Read the model definition and answer for the solid it produces. Units are mm, in the model's axes. Face numbers are marked on the shaded views. A direction names the side the tool comes from. Give positions to 0.01 mm unless a question says otherwise; leave off trailing zeros. Loops run counter-clockwise (first coordinate to the right, second up) from the corner with the lowest first, then second, coordinate; pieces in that order, holes last.
(1) Find section B-B, the plane z = 4.5. Write down the section's boundary in (x, y).
(2) Straight lines are drawn through the part: probe 1 along X at (y, z) = (-3.75, -0.5); probe 2 along Z at (x, y) = (-9.5, -4); probe 3 along Y at (x, z) = (-8.5, -2.25). For each, find the intervals that lie inside material, in ascending order.
(3) Each of these flat-tipped pins is pushed along its axis until it touches: P1, Ø0.8, axis at x = -17.375, z = 7.375, coming from the +Y side (3 decimals); P2, Ø1.8, axis at x = -18, z = 7, coming from the -Y side; P3, Ø9, axis at x = 9, z = 0.5, coming from the +Y side; P4, Ø0.5, axis at y = -6.5, z = -8.5, coming from the -X side. Where does it stop, or does it pass through?
(4) Find section A-A, the plane x = -9. Write down the section's boundary in (y, z).
(5) Find section C-C, the plane y = -3.5. Write down the section's boundary in (x, z) (3 decimals).
(6) Determine the mould class of the marked faces 3, 4 and 5 for opening direction Z: pulls with the +Z half, pulls with the -Z half, needs draft (parallel to the pull), parting line crosses it, or undercut.
(7) Which of the six approach directions +Z, -Z, +X, -X, +Y, -Y give full straight-line access (tool end or side, diameter ignored) to the marked faces 1 and 2?
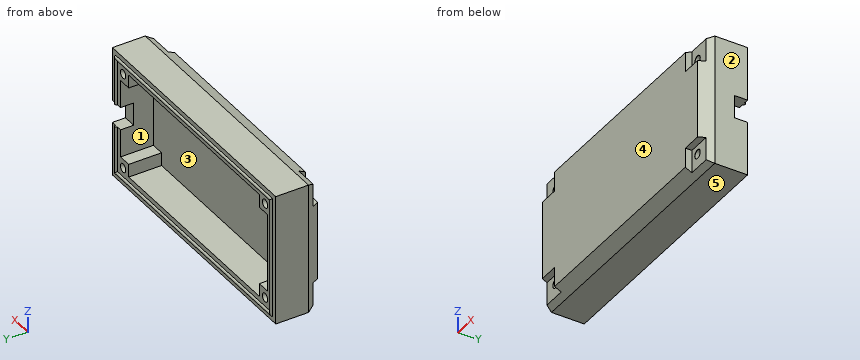
```python
from build123d import *

# Parameters (mm, degrees)
SCHIZZO2_W                     = 40
SCHIZZO2_H                     = 20
ESTRUSIONE_ESTRUSIONE1_DEPTH   = 7
TAGLIO_ESTRUSIONE1_DEPTH       = 5
SMUSSO1_SIZE                   = 1
SMUSSO1_SIZE2                  = 2
SCHIZZO6_W                     = 4
SCHIZZO6_H                     = 4
TAGLIO_ESTRUSIONE2_DEPTH       = 1
FORO_PER_VITE_M1_1_D           = 1.3
FORO_PER_VITE_M1_1_CSINK_D     = 1.35
FORO_PER_VITE_M1_1_CSINK_ANGLE = 90
SPECCHIA2_COPY_1_D             = 1.3
SPECCHIA2_COPY_1_CSINK_D       = 1.35
SPECCHIA2_COPY_1_CSINK_ANGLE   = 90
SCHIZZO14_W                    = 3.5
SCHIZZO14_H                    = 4
TAGLIO_ESTRUSIONE3_DEPTH       = 1
TAGLIO_ESTRUSIONE3_DEPTH_BACK  = 3


with BuildPart() as part:
    # Schizzo2 → Estrusione-Estrusione1 (new body)
    with BuildSketch(Plane(origin=(0, 0, 0), x_dir=(1, 0, 0), z_dir=(0, 1, 0))):
        Rectangle(SCHIZZO2_W, SCHIZZO2_H)
    extrude(amount=-ESTRUSIONE_ESTRUSIONE1_DEPTH)

    # Schizzo3 → Taglio-Estrusione1 (cut)
    with BuildSketch(Plane(origin=(0, 0, 0), x_dir=(1, 0, 0), z_dir=(0, 1, 0))):
        Polygon((-16, 8), (16, 8), (16, 6), (18, 6), (18, -6), (16, -6), (16, -8), (-16, -8), (-16, -6), (-18, -6), (-18, 6), (-16, 6), align=None)
    extrude(amount=-TAGLIO_ESTRUSIONE1_DEPTH, mode=Mode.SUBTRACT)

    # Sweep1: sweep along a path in Schizzo5
    with BuildLine(Plane(origin=(0, 0, 0), x_dir=(1, 0, 0), z_dir=(0, 1, 0))) as sweep1_path:
        Line((19, -9), (-19, -9))
        Line((-19, -9), (-19, 9))
        Line((-19, 9), (19, 9))
        Line((19, 9), (19, -9))
    # Schizzo4 → Sweep1 (sweep)
    with BuildSketch(Plane.XY):
        with BuildLine():
            Line((-18.75, 0), (-19.25, 0))
            ThreePointArc((-19.25, 0), (-19, 0.25), (-18.75, 0))
        make_face()
    sweep(path=sweep1_path.line, transition=Transition.RIGHT)

    # Smusso1
    smusso1_edges = [part.edges().sort_by_distance(p)[0] for p in [
        (20, -7, 0),
        (0, -7, -10),
        (-20, -7, 0),
        (0, -7, 10),
    ]]
    smusso1_side = [part.faces().sort_by_distance(p)[0] for p in [
        (0, -7, 0),
    ]]
    chamfer(smusso1_edges, length=SMUSSO1_SIZE, length2=SMUSSO1_SIZE2, reference=smusso1_side[0])

    # Schizzo6 → Taglio-Estrusione2 (cut)
    with BuildSketch(Plane.XZ.offset(7)):
        with Locations((-18, 8)):
            Rectangle(SCHIZZO6_W, SCHIZZO6_H)
        with Locations((18, 8)):
            Rectangle(SCHIZZO6_W, SCHIZZO6_H)
        with Locations((18, -8)):
            Rectangle(SCHIZZO6_W, SCHIZZO6_H)
        with Locations((-18, -8)):
            Rectangle(SCHIZZO6_W, SCHIZZO6_H)
    extrude(amount=-TAGLIO_ESTRUSIONE2_DEPTH, mode=Mode.SUBTRACT)

    # Foro per Vite M1-1 (through all)
    with Locations(Plane(origin=(0, -6, 0), x_dir=(-1, 0, 0), z_dir=(0, -1, 0))):
        with Locations((-17.375, 7.375)):
            foro_per_vite_m1_1 = CounterSinkHole(FORO_PER_VITE_M1_1_D / 2, FORO_PER_VITE_M1_1_CSINK_D / 2, counter_sink_angle=FORO_PER_VITE_M1_1_CSINK_ANGLE)

    # Specchia1: Foro per Vite M1-1 across plane
    add(foro_per_vite_m1_1.mirror(Plane(origin=(0, 0, 0), x_dir=(0, 0, 1), z_dir=(1, 0, 0))), mode=Mode.SUBTRACT)

    # Specchia2: Foro per Vite M1-1 across plane
    add(foro_per_vite_m1_1.mirror(Plane.XY), mode=Mode.SUBTRACT)

    # Specchia2 copy 1 (through all)
    with Locations(Plane.XZ.offset(6)):
        with Locations((-17.375, 7.375)):
            CounterSinkHole(SPECCHIA2_COPY_1_D / 2, SPECCHIA2_COPY_1_CSINK_D / 2, counter_sink_angle=SPECCHIA2_COPY_1_CSINK_ANGLE)

    # Schizzo14 → Taglio-Estrusione3 (cut, two sides)
    with BuildSketch(Plane(origin=(20, 0, 0), x_dir=(0, 0, -1), z_dir=(1, 0, 0))) as taglio_estrusione3_sk:
        Rectangle(SCHIZZO14_W, SCHIZZO14_H)
    extrude(amount=TAGLIO_ESTRUSIONE3_DEPTH, mode=Mode.SUBTRACT)
    extrude(taglio_estrusione3_sk.sketch, amount=-TAGLIO_ESTRUSIONE3_DEPTH_BACK, mode=Mode.SUBTRACT)


solid = part.part
```
Entries:
1. outline: (-20, -5) - (-19, -7) - (19, -7) - (20, -5) - (20, 0) - (19.25, 0) arc R0.25 ccw to (18.75, 0) - (18, 0) - (18, -5) - (-18, -5) - (-18, 0) - (-18.75, 0) arc R0.25 ccw to (-19.25, 0) - (-20, 0) - close
2. probe 1: x = -20 to -18, 18 to 20
2. probe 2: z = -10 to -8, 8 to 10
2. probe 3: y = -7 to -5
3. P1: passes through
3. P2: stops at y = -6
3. P3: stops at y = -5
3. P4: stops at x = -16
4. outline: (-7, -9) - (-5, -10) - (0, -10) - (0, -9.25) arc R0.25 ccw to (0, -8.75) - (0, -8) - (-5, -8) - (-5, 8) - (0, 8) - (0, 8.75) arc R0.25 ccw to (0, 9.25) - (0, 10) - (-5, 10) - (-7, 9) - close
5. outline: (-20, -10) - (20, -10) - (20, 10) - (-20, 10) - close; hole circle Ø1.3 at (-17.375, -7.375); hole circle Ø1.3 at (-17.375, 7.375); hole (-18, -6) - (-16, -6) - (-16, -8) - (16, -8) - (16, -6) - (18, -6) - (18, 6) - (16, 6) - (16, 8) - (-16, 8) - (-16, 6) - (-18, 6) - close; hole circle Ø1.3 at (17.375, -7.375); hole circle Ø1.3 at (17.375, 7.375)
6. face 3: undercut
6. face 4: needs draft
6. face 5: pulls with the -Z half
7. face 1: +Y
7. face 2: +Z, -Z, +X, +Y, -Y
